Check sheet for the drawn part. Datum: minimum x, y, z corner. Units: mm. A direction names the side the tool comes from. Round coordinates to 2 decimals unless told otherwise and drop trailing zeros. Order: outer loops, then holes, each group sorted by start corner. A loop starts at its lowest first (then second) coordinate and runs counter-clockwise, first axis right, second up. Notation, with made-up numbers: (-11.5, 11) -> (29.5, 11) arc R38 cw to (29.5, 50) -> close; hole circle Ø7 at (-37.5, 71). An arc over 180 degrees is marked (long way). Use CSV: the item, a comma, the result in double quotes.
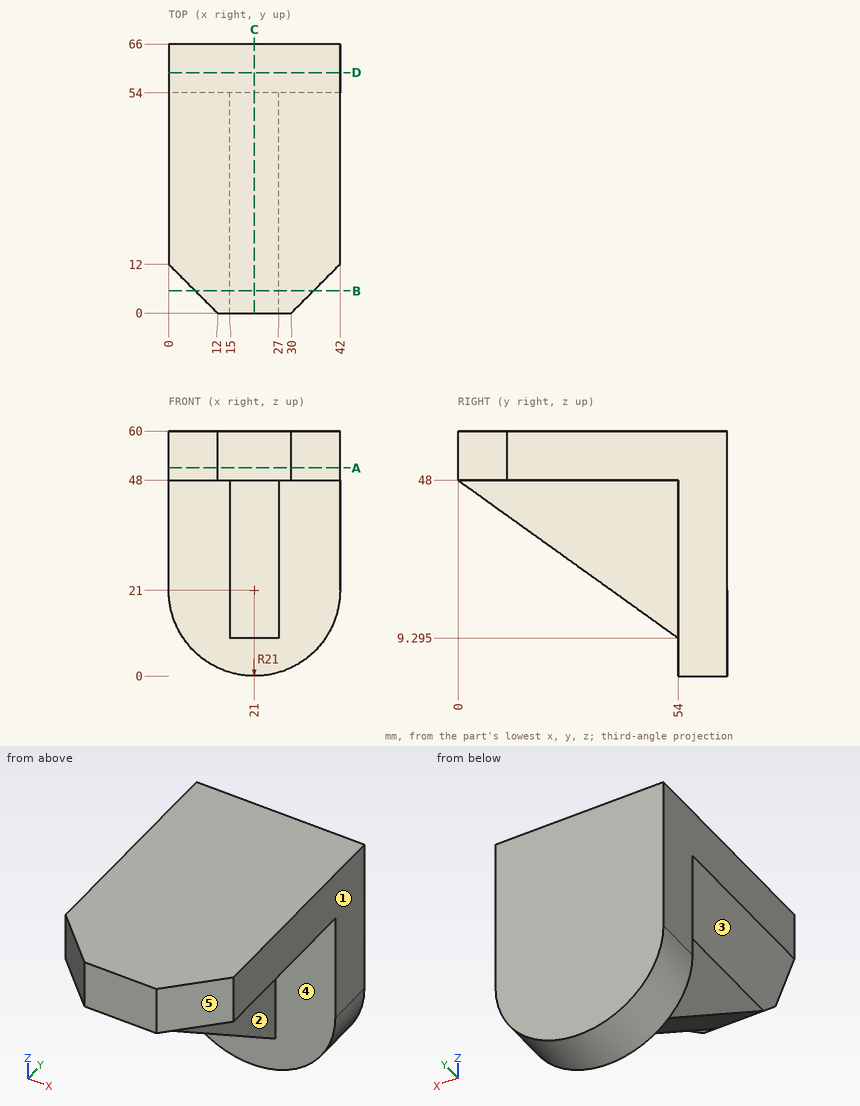
Q1. Access from +Z, -Z, +X, -X, +Y, -Y to the whole of each face (thin tool, end or side, straight path). Record for the marked faces 1, 2, 3, 4 and 5.
Result sheet:
face 1,"+Z, -Z, +X, +Y, -Y"
face 2,"-Z, +X, -Y"
face 3,"-Z, -X, -Y"
face 4,"-Z, -Y"
face 5,"+Z, -Z, +X, -Y"
Q2. Sectioned sample at B-B, the plane y = 5.5. Enter the section's corners in (x, z), then the cut area to 3 significant figures.
Result sheet:
outline,"(6.5, 48) -> (15, 48) -> (15, 44.06) -> (27, 44.06) -> (27, 48) -> (35.5, 48) -> (35.5, 60) -> (6.5, 60) -> close"
area,"395 mm^2"
Q3. Sectioned sample at A-A, the plane z = 51. Enter the section's corners in (x, y).
Result sheet:
outline,"(0, 12) -> (12, 0) -> (30, 0) -> (42, 12) -> (42, 66) -> (0, 66) -> close"
Q4. Scan lines: L1, parallel to X at y = 8, z = 47.5; L2, parallel to Z at x = 2.5, y = 15; L3, parallel to Y at x = 22.5, z = 5. Record each from-to range of solid material in increasing order.
Result sheet:
L1,"x = 15 to 27"
L2,"z = 48 to 60"
L3,"y = 54 to 66"
Q5. Sectioned sample at D-D, the plane y = 59. Enter the section's corners in (x, z).
Result sheet:
outline,"(0, 21) arc R21 ccw to (42, 21) -> (42, 60) -> (0, 60) -> close"
Q6. Go/stop test with flat-tipped pins: pin 1 (1.5 mm diameter, centred on x = 19, y = 9.5, fed in from -Z); pin 2 (10 mm diameter, centred on x = 28.5, y = 54, fed in from -Z); pin 3 (2 mm diameter, centred on x = 24, z = 33, fed in from -Y). Record where each tip stops, or that it passes through.
Result sheet:
pin 1,"stops at z = 40.65"
pin 2,"stops at z = 0.15"
pin 3,"stops at y = 19.53"
Q7. Sectioned sample at C-C, the plane x = 21. Enter the section's corners in (y, z) (3 decimals), then the cut area to 3 significant figures.
Result sheet:
outline,"(0, 48) -> (54, 9.295) -> (54, 0) -> (66, 0) -> (66, 60) -> (0, 60) -> close"
area,"2,410 mm^2"
